```python
from build123d import *

# Parameters (mm, degrees)
F1_DEPTH = 44.45
F2_R     = 4
F3_DEPTH = 8
F4_R     = 4
F5_DEPTH = 8
F7_DEPTH = 3
F9_DEPTH = 3


with BuildPart() as f1:
    # F0 (on Top) → F1 (new body)
    with BuildSketch(Plane.XY):
        with BuildLine():
            Line((8, 44.45), (0, 44.45))
            Line((0, 44.45), (0, 1))
            ThreePointArc((0, 1), (0.292893, 0.292893), (1, 0))
            Line((1, 0), (44.45, 0))
            Line((44.45, 0), (44.45, 8))
            Line((44.45, 8), (13, 8))
            ThreePointArc((13, 8), (9.464466, 9.464466), (8, 13))
            Line((8, 13), (8, 44.45))
        make_face()
    extrude(amount=F1_DEPTH)

    # F2 (on face) → F3 (cut, through all)
    with BuildSketch(Plane.YZ.offset(8)):
        with Locations((25.4, 22.225)):
            Circle(F2_R)
    extrude(amount=-F3_DEPTH, mode=Mode.SUBTRACT)

    # F4 (on face) → F5 (cut, through all)
    with BuildSketch(Plane.XZ):
        with Locations((25.4, 22.225)):
            Circle(F4_R)
    extrude(amount=-F5_DEPTH, mode=Mode.SUBTRACT)

    # F6 (on face) → F7 (cut)
    with BuildSketch(Plane.YZ.offset(8)):
        Polygon((25.4, 14.225812), (32.3275, 18.225406), (32.3275, 26.224594), (25.4, 30.224188), (18.4725, 26.224594), (18.4725, 18.225406), align=None)
    extrude(amount=-F7_DEPTH, mode=Mode.SUBTRACT)

    # F8 (on face) → F9 (cut)
    with BuildSketch(Plane(origin=(0, 8, 0), x_dir=(-1, 0, 0), z_dir=(0, 1, 0))):
        Polygon((-25.4, 30.224188), (-32.3275, 26.224594), (-32.3275, 18.225406), (-25.4, 14.225812), (-18.4725, 18.225406), (-18.4725, 26.224594), align=None)
    extrude(amount=-F9_DEPTH, mode=Mode.SUBTRACT)


solid = f1.part
```
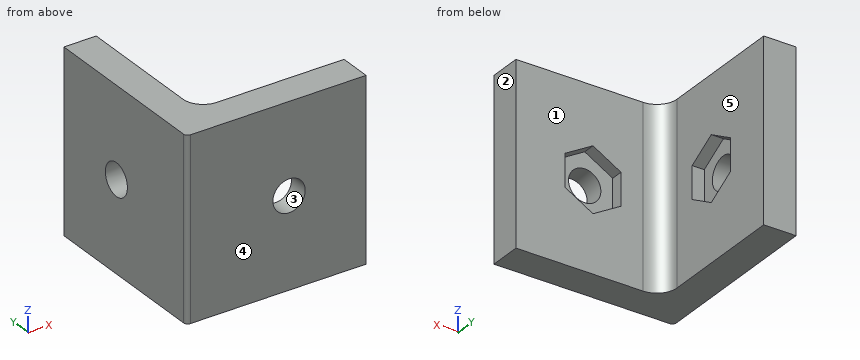
The model under review builds one solid part; all positions refer to its coordinate system, in mm. Face numbers are marked on the shaded views. A direction names the side the tool comes from. Round coordinates to 2 decimals unless told otherwise and drop trailing zeros. Loops run counter-clockwise (first coordinate to the right, second up) from the corner with the lowest first, then second, coordinate; pieces in that order, holes last. Notation, with made-up numbers: (2, 36) -> (30, 36) arc R16 ccw to (30, 46) -> close; hole circle Ø8 at (56.25, 6.25). An arc over 180 degrees is marked (long way). Answer as a JSON object with one key per item and string values. Group by question number.
1) For the marked faces 4 and 5, list the 3-axis set-ups (+Z, -Z, +X, -X, +Y, -Y) from which the entire face can be reached by the end or side of a thin tool; tool diameter is ignored.
2) For pin 1 Ø4 at (y, z) = (14.5, 18) entering from +X; pin 2 Ø13 at (x, z) = (25.4, 22.225) entering from -Y; pin 3 Ø12 at (x, z) = (38.5, 7.5) entering from +Y, all flat-tipped, find the tip position at first contact; note any pin that passes through.
3) Mouldability with a two-part tool opening along X and no side actions: class the marked faces 1, 2 and 3 as released by +X, released by -X, zero draft, split by the parting line, or undercut.
4) For line 1 (Z direction, x = 25.4, y = 2.45) (3 decimals); line 2 (Y direction, x = 42.5, z = 10), list the stretches that pass through material, from the lowest coordinate up. Write a range as [from, to].
5) We need section B-B on z = 37.5. Write out the cut boundary in (x, y), then the cut area to 3 significant figures.
6) We need section D-D on y = 31.5. Write out the cut boundary in (x, z), then the cut area to 3 significant figures.
7) We need section A-A on x = 24. Write out the cut boundary in (y, z).
8) We need section C-C on x = 37. Write out the cut boundary in (y, z), then the cut area to 3 significant figures.
Result set:
{
 "1": {"face 4": "+Z, -Z, +X, -X, -Y", "face 5": "+Z, -Z, +X, +Y"},
 "2": {"pin 1": "x = 8.03", "pin 2": "y = 0", "pin 3": "y = 8"},
 "3": {"face 1": "zero draft", "face 2": "released by +X", "face 3": "undercut"},
 "4": {"line 1": "[0, 18.225], [26.225, 44.45]", "line 2": "[0, 8]"},
 "5": {"outline": "(0, 1) arc R1 ccw to (1, 0) -> (44.45, 0) -> (44.45, 8) -> (13, 8) arc R5 cw to (8, 13) -> (8, 44.45) -> (0, 44.45) -> close", "area": "652 mm²"},
 "6": {"outline": "(0, 0) -> (8, 0) -> (8, 17.75) -> (5, 17.75) -> (5, 26.7) -> (8, 26.7) -> (8, 44.45) -> (0, 44.45) -> close", "area": "329 mm²"},
 "7": {"outline": "(0, 0) -> (8, 0) -> (8, 15.03) -> (5, 15.03) -> (5, 18.48) -> (0, 18.48) -> close; (0, 25.97) -> (5, 25.97) -> (5, 29.42) -> (8, 29.42) -> (8, 44.45) -> (0, 44.45) -> close"},
 "8": {"outline": "(0, 0) -> (8, 0) -> (8, 44.45) -> (0, 44.45) -> close", "area": "356 mm²"}
}
